Here's how the part is built. I have some questions about the finished solid (model axes, mm). Face numbers are marked on the shaded views. A direction names the side the tool comes from. Round coordinates to 2 decimals unless told otherwise and drop trailing zeros. Order: outer loops, then holes, each group sorted by start corner. A loop starts at its lowest first (then second) coordinate and runs counter-clockwise, first axis right, second up.
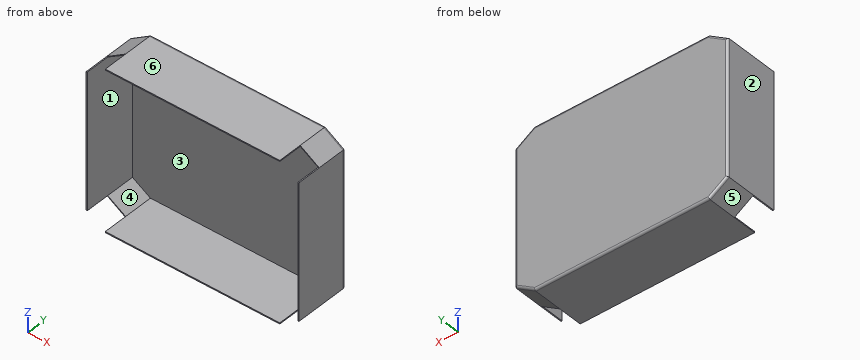
```python
from build123d import *

# Parameters (mm, degrees)
SKETCH1_W             = 210.556721652
SKETCH1_H             = 1.27
BOSS_EXTRUDE1_DEPTH   = 29.21
SKETCH1_W_2           = 1.27
SKETCH1_H_2           = 163.559236
BOSS_EXTRUDE1_2_DEPTH = 29.21
BOSS_EXTRUDE1_3_DEPTH = 29.21
BOSS_EXTRUDE1_4_DEPTH = 29.21
BOSS_EXTRUDE2_DEPTH   = 35.56
BOSS_EXTRUDE3_DEPTH   = 1.27
FILLET1_R             = 2.54


with BuildPart() as part:
    # Sketch1 → Boss-Extrude1 (new body)
    with BuildSketch(Plane(origin=(0, 0, 0), x_dir=(1, 0, 0), z_dir=(0, 1, 0))):
        with Locations((0, -95.885)):
            Rectangle(SKETCH1_W, SKETCH1_H)
    extrude(amount=BOSS_EXTRUDE1_DEPTH)



with BuildPart() as body_2:
    # Sketch1 → Boss-Extrude1 2 (new body)
    with BuildSketch(Plane(origin=(0, 0, 0), x_dir=(1, 0, 0), z_dir=(0, 1, 0))):
        with Locations((-127.635, 0)):
            Rectangle(SKETCH1_W_2, SKETCH1_H_2)
    extrude(amount=BOSS_EXTRUDE1_2_DEPTH)


with BuildPart() as body_3:
    # Sketch1 → Boss-Extrude1 3 (new body)
    with BuildSketch(Plane(origin=(0, 0, 0), x_dir=(1, 0, 0), z_dir=(0, 1, 0))):
        with Locations((0, 95.885)):
            Rectangle(SKETCH1_W, SKETCH1_H)
    extrude(amount=BOSS_EXTRUDE1_3_DEPTH)


with BuildPart() as body_4:
    # Sketch1 → Boss-Extrude1 4 (new body)
    with BuildSketch(Plane(origin=(0, 0, 0), x_dir=(1, 0, 0), z_dir=(0, 1, 0))):
        with Locations((127.635, 0)):
            Rectangle(SKETCH1_W_2, SKETCH1_H_2)
    extrude(amount=BOSS_EXTRUDE1_4_DEPTH)


with BuildPart() as part_1:
    add(part.part)

    add(body_2.part)  # Boss-Extrude2 merges body 2

    add(body_3.part)  # Boss-Extrude2 merges body 3

    add(body_4.part)  # Boss-Extrude2 merges body 4
    # Sketch4 → Boss-Extrude2 (add)
    with BuildSketch(Plane(origin=(0, 29.21, 0), x_dir=(1, 0, 0), z_dir=(0, 1, 0))):
        Polygon((-128.27, 81.779618), (-105.278360826, 96.52), (105.278360826, 96.52), (128.27, 81.779618), (128.27, -81.779618), (105.278360826, -96.52), (-105.278360826, -96.52), (-128.27, -81.779618), align=None)
        Polygon((-127, 81.779618), (-105.278360826, 95.25), (105.278360826, 95.25), (127, 81.779618), (127, -81.779618), (105.278360826, -95.25), (-105.278360826, -95.25), (-127, -81.779618), align=None, mode=Mode.SUBTRACT)
    extrude(amount=BOSS_EXTRUDE2_DEPTH)

    # Sketch5 → Boss-Extrude3 (add)
    with BuildSketch(Plane(origin=(0, 64.77, 0), x_dir=(1, 0, 0), z_dir=(0, 1, 0))):
        Polygon((-128.27, 81.779618), (-105.278360826, 96.52), (105.278360826, 96.52), (128.27, 81.779618), (128.27, -81.779618), (105.278360826, -96.52), (-105.278360826, -96.52), (-128.27, -81.779618), align=None)
    extrude(amount=BOSS_EXTRUDE3_DEPTH)

    # Fillet1
    fillet1_edges = [part_1.edges().sort_by_distance(p)[0] for p in [
        (-128.27, 66.04, 0),
        (-116.774180413, 66.04, 89.149809),
        (0, 66.04, 96.52),
        (116.774180413, 66.04, 89.149809),
        (128.27, 66.04, 0),
        (116.774180413, 66.04, -89.149809),
        (0, 66.04, -96.52),
        (-116.774180413, 66.04, -89.149809),
    ]]
    fillet(fillet1_edges, radius=FILLET1_R)


solid = part_1.part
```
1. On a 3-axis mill with a long thin cutter (end or side, diameter ignored), from which of +Z, -Z, +X, -X, +Y, -Y can I reach the whole of each face in a straight line? I mean the marked faces 1 and 2. Say none if no direction works.
Evaluation:
face 1: -Y
face 2: +Z, -Z, -X, +Y, -Y
2. I'm going to push flat-ended pins straight in: P1, Ø12, axis at x = 111.5, z = -90.5, coming from the -Y side; P2, Ø1.4, axis at x = 127.5, y = 20, coming from the +Z side; P3, Ø1, axis at y = 14.5, z = 96, coming from the -X side. Where does each tip first touch, or does it pass through?
Evaluation:
P1: stops at y = 29.21
P2: stops at z = 81.78
P3: stops at x = -105.28
3. If we section it at A-A, the plane y = 44.5: Write out the boundary of the cut face in (x, z).
Evaluation:
outline: (-128.27, -81.78) - (-105.28, -96.52) - (105.28, -96.52) - (128.27, -81.78) - (128.27, 81.78) - (105.28, 96.52) - (-105.28, 96.52) - (-128.27, 81.78) - close; hole (-127, -81.78) - (-105.28, -95.25) - (105.28, -95.25) - (127, -81.78) - (127, 81.78) - (105.28, 95.25) - (-105.28, 95.25) - (-127, 81.78) - close
4. If we section it at B-B, the plane y = 19: Write out the boundary of the cut face in (x, z), and give its area (3 significant figures).
Evaluation:
outline: (-128.27, -81.78) - (-127, -81.78) - (-127, 81.78) - (-128.27, 81.78) - close; (-105.28, -96.52) - (105.28, -96.52) - (105.28, -95.25) - (-105.28, -95.25) - close; (-105.28, 95.25) - (105.28, 95.25) - (105.28, 96.52) - (-105.28, 96.52) - close; (127, -81.78) - (128.27, -81.78) - (128.27, 81.78) - (127, 81.78) - close
area: 950 mm2
5. If we section it at C-C, the plane x = 30: Write out the boundary of the cut face in (y, z), and give its area (3 significant figures).
Evaluation:
outline: (0, -96.52) - (63.5, -96.52) arc R2.54 ccw to (66.04, -93.98) - (66.04, 93.98) arc R2.54 ccw to (63.5, 96.52) - (0, 96.52) - (0, 95.25) - (64.77, 95.25) - (64.77, -95.25) - (0, -95.25) - close
area: 407 mm2
6. I need wall thicknesses on probe 1 along Z at (x, y) = (83.5, 43.5); probe 2 along X at (y, z) = (58.5, 61.5); probe 3 along Y at (x, z) = (-29, 70). Which ranges of each line are inside material? Lowest first, please.
Evaluation:
probe 1: z = -96.52 to -95.25, 95.25 to 96.52
probe 2: x = -128.27 to -127, 127 to 128.27
probe 3: y = 64.77 to 66.04
7. If we section it at D-D, the plane z = -30.5: Write out the boundary of the cut face in (x, y), and give its area (3 significant figures).
Evaluation:
outline: (-128.27, 0) - (-127, 0) - (-127, 64.77) - (127, 64.77) - (127, 0) - (128.27, 0) - (128.27, 63.5) arc R2.54 ccw to (125.73, 66.04) - (-125.73, 66.04) arc R2.54 ccw to (-128.27, 63.5) - close
area: 488 mm2
8. If we mould it in two halves opening along Z, with no side actions, what happens to the marked faces 3, 4, 5 and 6? For each: released by +Z, released by -Z, zero draft, split by the parting line, or undercut.
Evaluation:
face 3: undercut
face 4: undercut
face 5: released by -Z
face 6: released by +Z
